Check sheet for the modelled part. Datum: model origin and axes. Units: mm. A direction names the side the tool comes from. Give positions to 0.01 mm unless a question says otherwise; leave off trailing zeros. Loops run counter-clockwise (first coordinate to the right, second up) from the corner with the lowest first, then second, coordinate; pieces in that order, holes last. Notation, with made-up numbers: (-6, 89) -> (26, 89) arc R17 cw to (26, 109) -> close; hole circle Ø8 at (-22, 2). An arc over 180 degrees is marked (long way). Answer as CSV lines item,"result". Start each with the question number.
(1) Access from +Z, -Z, +X, -X, +Y, -Y to the whole of each face (thin tool, end or side, straight path). Record for faces 4 (the face through (214.636, -213.63, 295.8)), 5 (the face through (250, -3, 296)).
(2) Material ranges on line 1 (X direction, y = -169.5, z = 371); line 2 (Y direction, x = -91.5, z = 257); line 3 (Y direction, x = -210, z = 436), recorded low to high. Write a range as from..to.
(3) Section check B-B on z = 349. Enter the section's corners in (x, y).
(4) Release check for a two-part mould opening along X. For faces 1 (the face through (214.32, 213.96, 295.8)), 2 (the face through (-250, -3, 296)), 3 (the face through (-223, 1, 0)) record: pulls with the +X half, pulls with the -X half, needs draft (parallel to the pull), parting line crosses it, or undercut.
(5) Section check A-A on y = 65. Enter the section's corners in (x, z).
(6) Section check C-C on x = -128. Enter the section's corners in (y, z).
from build123d import *

# Parameters (mm, degrees)
F0_W     = 500
F0_H     = 500
F1_DEPTH = 600


with BuildPart() as f1:
    # F0 (on Top) → F1 (new body)
    with BuildSketch(Plane.XY):
        Rectangle(F0_W, F0_H)
        with BuildLine():
            ThreePointArc((-200.145707391, 219.9994692269), (-200.000026529, 220), (-199.8543456655, 219.9994696133))
            Line((-199.8543456655, 219.9994696133), (199.999973471, 220))
            ThreePointArc((199.999973471, 220), (214.4809440479, 213.7950084988), (219.9764733348, 199.0301994505))
            Line((219.9764733348, 199.0301994505), (219.9764733348, -199.0301994505))
            ThreePointArc((219.9764733348, -199.0301994505), (214.480905162, -213.7950493181), (199.9998607178, -219.9999999995))
            Line((199.9998607178, -219.9999999995), (-199.6663459368, -219.9972166805))
            ThreePointArc((-199.6663459368, -219.9972166805), (-200.0001392822, -219.9999999995), (-200.3339325887, -219.9972120313))
            ThreePointArc((-200.3339325887, -219.9972120313), (-214.0088543508, -214.2741724726), (-219.9874282617, -200.7090214974))
            ThreePointArc((-219.9874282617, -200.7090214974), (-220, -200), (-219.9874282617, -199.2909785026))
            Line((-219.9874282617, -199.2909785026), (-219.9874282617, 199.2909785026))
            ThreePointArc((-219.9874282617, 199.2909785026), (-220, 200), (-219.9874282617, 200.7090214974))
            ThreePointArc((-219.9874282617, 200.7090214974), (-213.941525426, 214.3399396371), (-200.145707391, 219.9994692269))
        make_face(mode=Mode.SUBTRACT)
    extrude(amount=F1_DEPTH)


solid = f1.part
Working result:
1,face 4,"+Z, -Z"
1,face 5,"+Z, -Z, +X, +Y, -Y"
2,line 1,"x = -250..-219.99, 219.98..250"
2,line 2,"y = -250..-220, 220..250"
2,line 3,"y = -250..-217.32, 217.32..250"
3,outline,"(-250, -250) -> (250, -250) -> (250, 250) -> (-250, 250) -> close; hole (-219.99, -199.29) arc R20 ccw to (-199.67, -220) -> (200, -220) arc R20 ccw to (219.98, -199.03) -> (219.98, 199.03) arc R20 ccw to (200, 220) -> (-199.85, 220) arc R20 ccw to (-219.99, 199.29) -> close"
4,face 1,"undercut"
4,face 2,"pulls with the -X half"
4,face 3,"needs draft"
5,outline,"(-250, 0) -> (-219.99, 0) -> (-219.99, 600) -> (-250, 600) -> close; (219.98, 0) -> (250, 0) -> (250, 600) -> (219.98, 600) -> close"
6,outline,"(-250, 0) -> (-220, 0) -> (-220, 600) -> (-250, 600) -> close; (220, 0) -> (250, 0) -> (250, 600) -> (220, 600) -> close"
